from build123d import *

# Parameters (mm, degrees)
SKETCH014_W         = 85
SKETCH014_H         = 245
PAD009_DEPTH        = 20
SKETCH015_R         = 7.5
PAD010_DEPTH        = 10
PAD011_DEPTH        = 25
SKETCH017_R         = 2.1
HOLE005_DEPTH       = 25.001
HOLE006_D           = 5.8
HOLE006_DEPTH       = 25
HOLE006_CBORE_D     = 13
HOLE006_CBORE_DEPTH = 6.4


with BuildPart() as part:
    # Sketch014 → Pad009 (new body)
    with BuildSketch(Plane.XZ.offset(25)):
        with Locations((87.5, 127.5)):
            Rectangle(SKETCH014_W, SKETCH014_H)
    extrude(amount=PAD009_DEPTH)

    # Sketch015 → Pad010 (join)
    with BuildSketch(Plane.XZ.offset(40)):
        with Locations((77.5, 230)):
            Circle(SKETCH015_R)
        with Locations((120, 218)):
            Circle(SKETCH015_R)
        with Locations((55, 135)):
            Circle(SKETCH015_R)
        with Locations((42.5, 42.5)):
            Circle(SKETCH015_R)
        with Locations((81, 75)):
            Circle(SKETCH015_R)
    extrude(amount=PAD010_DEPTH)

    # Sketch016 → Pad011 (join)
    with BuildSketch(Plane.XY.offset(30)):
        Polygon((35, -40), (45, -30), (45, -45), (35, -45), align=None)
    extrude(amount=PAD011_DEPTH)

    # Sketch017 → Hole005 (cut, through all)
    with BuildSketch(Plane.XZ.offset(50)):
        with Locations((77.5, 230)):
            Circle(SKETCH017_R)
        with Locations((120, 218)):
            Circle(SKETCH017_R)
        with Locations((55, 135)):
            Circle(SKETCH017_R)
        with Locations((42.5, 42.5)):
            Circle(SKETCH017_R)
        with Locations((81, 75)):
            Circle(SKETCH017_R)
    extrude(amount=-HOLE005_DEPTH, mode=Mode.SUBTRACT)

    # Hole006
    with Locations(Plane.XZ.offset(45)):
        with Locations((60, 230), (60, 190), (60, 150), (60, 110), (60, 70), (60, 30)):
            CounterBoreHole(HOLE006_D / 2, HOLE006_CBORE_D / 2, HOLE006_CBORE_DEPTH, depth=HOLE006_DEPTH)


solid = part.part
The model under review builds one solid part; all positions refer to its coordinate system, in mm. A direction names the side the tool comes from. Coordinates: 2 decimals unless noted, no trailing zeros. Write each loop counter-clockwise with the first axis right and the second up, starting at its lowest first coordinate (ties: lowest second). Pieces come first, ordered by that corner, then holes. Notation, with made-up numbers: M -4,-8.5 L 42,-8.5 A15 ccw 42,6.5 Z; hole C 48.25,75.5 d8. An arc over 180 degrees is marked long. Put each result on its own line as item: value.
1) Draft analysis for pull direction X (two halves, no side actions). For faces 3 (the flat face through (35, -43, 42)), 4 (the cylindrical face through (58.66, -31.7, 67.43)), 5 (the cylindrical face through (66.2, -41.84, 31.95)), 6 (the flat face through (57, -50, 133)), state which applies: released by +X, released by -X, zero draft, split by the parting line, or undercut.
Computed:
face 3: released by -X
face 4: undercut
face 5: undercut
face 6: zero draft
2) Add section A-A on y = -27.75. State how many separate pieces and enclosed holes the cut face has, then the cut area to 3 significant figures.
Computed:
separate pieces: 1
enclosed holes: 10
area: 20,600 mm2
3) Add section C-C on z = 199. Give the boundary of the cut face in (x, y).
Computed:
outline: M 45,-45 L 130,-45 L 130,-25 L 45,-25 Z
4) Clearance check with flat-ended pins moving along their axes: pin 1 Ø6.5 at (x, z) = (81, 75) entering from +Y; pin 2 Ø4 at (x, z) = (60, 32) entering from -Y; pin 3 Ø1 at (x, z) = (93, 140) entering from -Y; pin 4 Ø3.5 at (x, z) = (60, 110) entering from -Y. State where each tip first meets the part, or that it passes through.
Computed:
pin 1: stops at y = -25
pin 2: stops at y = -38.6
pin 3: stops at y = -45
pin 4: passes through
5) Wall thickness on probe 1 along Z at (x, y) = (77.5, -41.75); probe 2 along Z at (x, y) = (81, -38.75); probe 3 along X at (y, z) = (-44.25, 135): over which ranges is each line inside the solid? List them lowest first. Write a range as [from, to].
Computed:
probe 1: z = [5, 227.9], [232.1, 250]
probe 2: z = [5, 72.9], [77.1, 250]
probe 3: x = [45, 52.9], [57.1, 130]
6) For faces 1 (the flat face through (87, -35, 5)), 2 (the flat face through (61, -38.6, 27)), list the 3-axis set-ups (+Z, -Z, +X, -X, +Y, -Y) from which the entire face can be reached by the end or side of a thin tool; tool diameter is ignored.
Computed:
face 1: -Z, +X, -X, +Y, -Y
face 2: -Y
7) Add section D-D on x = 96.5. Give the boundary of the cut face in (y, z), then the cut area to 3 significant figures.
Computed:
outline: M -45,5 L -25,5 L -25,250 L -45,250 Z
area: 4,900 mm2
